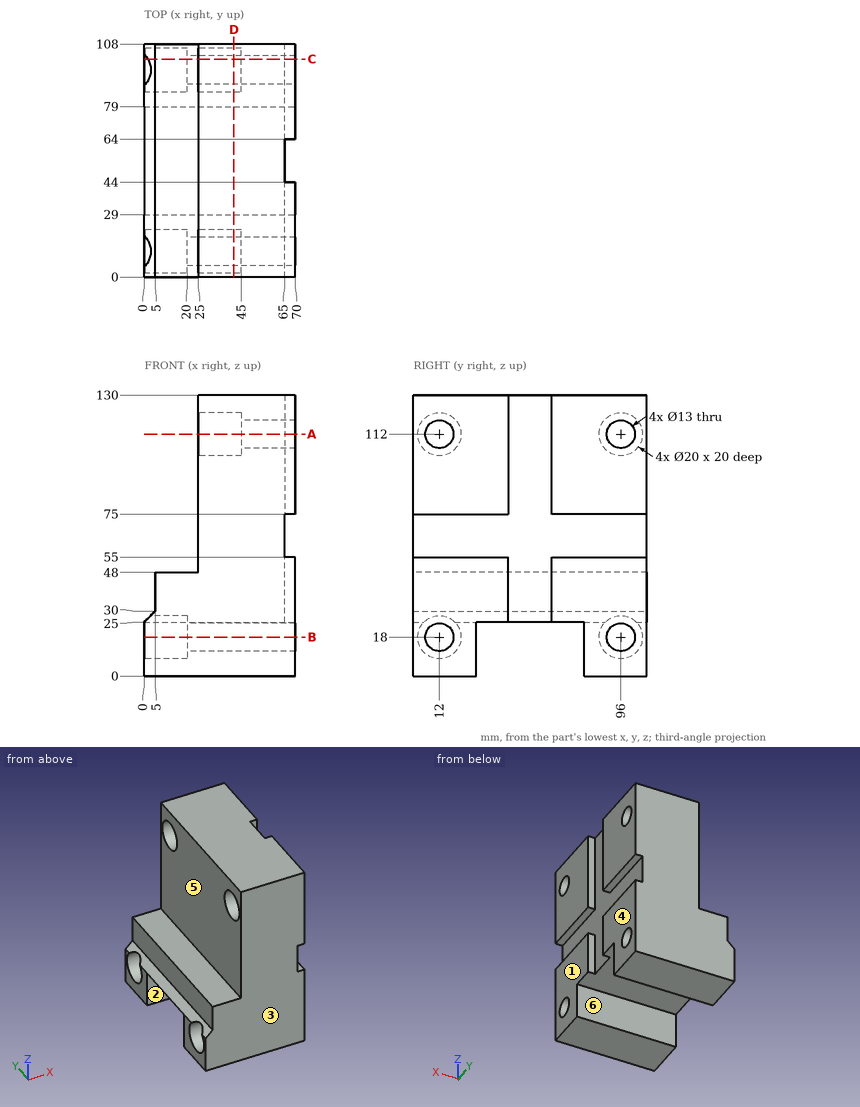
Part print with two shaded views. Sizes in mm from the minimum x, y, z corner. A direction names the side the tool comes from. Round coordinates to 2 decimals unless told otherwise and drop trailing zeros. Order: outer loops, then holes, each group sorted by start corner. A loop starts at its lowest first (then second) coordinate and runs counter-clockwise, first axis right, second up. Notation, with made-up numbers: M -18,56.5 L 22,56.5 A15 ccw 22,74.5 Z; hole C -15.5,48 d4. An arc over 180 degrees is marked long. Use CSV: the item, a comma, the result in double quotes.
Item 1: Saw through at A-A (z = 112). List the corners of the cut face in (x, y).
Worked answers:
outline,"M 25,0 L 70,0 L 70,5.5 L 45,5.5 L 45,2 L 25,2 Z; M 25,22 L 45,22 L 45,18.5 L 70,18.5 L 70,44 L 65,44 L 65,64 L 70,64 L 70,89.5 L 45,89.5 L 45,86 L 25,86 Z; M 25,106 L 45,106 L 45,102.5 L 70,102.5 L 70,108 L 25,108 Z"
Item 2: Which spindle directions (+Z, -Z, +X, -X, +Y, -Y) get a long thin tool onto all of the face, cutting with end or side? Do the marked faces 4, 5 and 6. Say none if no direction does.
Worked answers:
face 4,"+Z, -Z, +X, +Y, -Y"
face 5,"+Z, -X, +Y, -Y"
face 6,"-Z, +X, -X"
Item 3: Saw through at B-B (z = 18). List the corners of the cut face in (x, y).
Worked answers:
outline,"M 0,0 L 70,0 L 70,5.5 L 20,5.5 L 20,2 L 0,2 Z; M 0,22 L 20,22 L 20,18.5 L 70,18.5 L 70,29 L 0,29 Z; M 0,79 L 70,79 L 70,89.5 L 20,89.5 L 20,86 L 0,86 Z; M 0,106 L 20,106 L 20,102.5 L 70,102.5 L 70,108 L 0,108 Z"
Item 4: Probe probe 1 along Z at (x, y) = (35, 12); probe 2 along Z at (x, y) = (62.5, 12); probe 3 along Y at (x, z) = (9, 18). List the from-to ranges inside material, lowest first.
Worked answers:
probe 1,"0 to 11.5, 24.5 to 102, 122 to 130"
probe 2,"0 to 11.5, 24.5 to 105.5, 118.5 to 130"
probe 3,"0 to 2, 22 to 29, 79 to 86, 106 to 108"
Item 5: Pull direction Y, two halves, no side cores. Call the marked faces 1, 2 and 3: released by +Y, released by -Y, zero draft, split by the parting line, or undercut.
Worked answers:
face 1,"zero draft"
face 2,"undercut"
face 3,"released by -Y"
Item 6: Pin check, flat tips, straight feed: pin 1 (1.5 mm diameter, centred on x = 58.5, z = 56, fed in from -Y); pin 2 (3 mm diameter, centred on x = 19.5, y = 33.5, fed in from -Z); pin 3 (5 mm diameter, centred on y = 93.5, z = 47.5, fed in from -X); pin 4 (6 mm diameter, centred on x = 13.5, y = 48, fed in from +Z). Stop position of each tip, or through.
Worked answers:
pin 1,"y = 0"
pin 2,"z = 25"
pin 3,"x = 5"
pin 4,"z = 48"
Item 7: Saw through at D-D (x = 41.5). List the corners of the cut face in (y, z).
Worked answers:
outline,"M 0,0 L 29,0 L 29,25 L 79,25 L 79,0 L 108,0 L 108,130 L 0,130 Z; hole C 12,112 d20; hole C 12,18 d13; hole C 96,112 d20; hole C 96,18 d13"
Item 8: Saw through at C-C (y = 101). List the corners of the cut face in (x, z), plus the area to 3 significant figures.
Worked answers:
outline,"M 0,0 L 70,0 L 70,13.85 L 20,13.85 L 20,9.34 L 0,9.34 Z; M 1.66,26.66 L 20,26.66 L 20,22.15 L 70,22.15 L 70,55 L 65,55 L 65,75 L 70,75 L 70,107.85 L 45,107.85 L 45,103.34 L 25,103.34 L 25,48 L 5,48 L 5,30 Z; M 25,120.66 L 45,120.66 L 45,116.15 L 70,116.15 L 70,130 L 25,130 Z"
area,"5,530 mm²"
